```python
from build123d import *

# Parameters (mm, degrees)
F0_W      = 126.2549012899
F0_H      = 84.0705931187
F1_DEPTH  = 10
F2_W      = 119.4519400597
F2_H      = 78.4470066428
F3_DEPTH  = 9
F6_R      = 2.7574274492
F6_R_2    = 3.0881184617
F6_R_3    = 2.9865161703
F7_DEPTH  = 9.5
F5_R      = 3.0287162896
F8_DEPTH  = 9.5
F4_R      = 3.8384708655
F9_DEPTH  = 9.5
F10_R     = 3.132111717
F10_R_2   = 2.9916448853
F10_R_3   = 3.0367007185
F10_R_4   = 2.8900379759
F11_DEPTH = 9.5
F13_R     = 3.0036385534
F13_R_2   = 2.9794176667
F13_R_3   = 3.6399459422
F13_R_4   = 3.1255773117
F14_DEPTH = 9.5
F12_R     = 3.2154485225
F12_R_2   = 2.6789056155
F12_R_3   = 3.0133824395
F12_R_4   = 3.8856724273
F15_DEPTH = 9.5
F16_R     = 3.6323450942
F16_R_2   = 3.9223279678
F17_DEPTH = 9.5


# Not quite as in the source:
# - a feature names something its author has since deleted; it is built from what else it names


with BuildPart() as f1:
    # F0 (on Top) → F1 (new body)
    with BuildSketch(Plane.XY):
        Rectangle(F0_W, F0_H)
    extrude(amount=-F1_DEPTH)

    # F2 (on Top) → F3 (cut)
    with BuildSketch(Plane.XY):
        Rectangle(F2_W, F2_H)
    extrude(amount=-F3_DEPTH, mode=Mode.SUBTRACT)

    # F6 (on Top) → F7 (cut)
    with BuildSketch(Plane.XY):
        with Locations((16.5214389563, -8.0118775368)):
            Circle(F6_R)
        with Locations((-16.615998, -8.0534629524)):
            Circle(F6_R_2)
        with Locations((-16.615998, 8.0431699753)):
            Circle(F6_R_3)
    extrude(amount=-F7_DEPTH, mode=Mode.SUBTRACT)

    # F5 (on Top) → F8 (cut)
    with BuildSketch(Plane.XY):
        with Locations((16.5819376707, 7.8347064555)):
            Circle(F5_R)
    extrude(amount=-F8_DEPTH, mode=Mode.SUBTRACT)

    # F4 (on Top) → F9 (cut)
    with BuildSketch(Plane.XY):
        Circle(F4_R)
    extrude(amount=-F9_DEPTH, mode=Mode.SUBTRACT)

    # F10 (on face) → F11 (cut)
    with BuildSketch(Plane.XY):
        with Locations((29.441639781, 19.3310081959)):
            Circle(F10_R)
        with Locations((29.7522768378, -19.6110159159)):
            Circle(F10_R_2)
        with Locations((-29.6404287219, -19.6110159159)):
            Circle(F10_R_3)
        with Locations((-29.5161753893, 19.5709131658)):
            Circle(F10_R_4)
    extrude(amount=-F11_DEPTH, mode=Mode.SUBTRACT)

    # F13 (on Top) → F14 (cut)
    with BuildSketch(Plane.XY):
        with Locations((-34.714885056, 0)):
            Circle(F13_R)
        with Locations((35.1781696081, 0)):
            Circle(F13_R_2)
        with Locations((-51.6325049102, 0)):
            Circle(F13_R_3)
        with Locations((51.6923218966, 0)):
            Circle(F13_R_4)
    extrude(amount=-F14_DEPTH, mode=Mode.SUBTRACT)

    # F12 (on Top) → F15 (cut)
    with BuildSketch(Plane.XY):
        with Locations((-51.8871918321, 32.8838564456)):
            Circle(F12_R)
        with Locations((-51.9447661936, -32.4058681726)):
            Circle(F12_R_2)
        with Locations((51.5429228544, -32.7062048018)):
            Circle(F12_R_3)
        with Locations((51.7358258367, 31.9894589484)):
            Circle(F12_R_4)
    extrude(amount=-F15_DEPTH, mode=Mode.SUBTRACT)

    # F16 (on Top) → F17 (cut)
    with BuildSketch(Plane.XY):
        with Locations((0, 25.2807121724)):
            Circle(F16_R)
        with Locations((0, -27.0220451057)):
            Circle(F16_R_2)
    extrude(amount=-F17_DEPTH, mode=Mode.SUBTRACT)


solid = f1.part
```
CAD build for the part. Positions are in the model's coordinates, mm. A direction names the side the tool comes from. Round coordinates to 2 decimals unless told otherwise and drop trailing zeros. Write each loop counter-clockwise with the first axis right and the second up, starting at its lowest first coordinate (ties: lowest second). Pieces come first, ordered by that corner, then holes.
Item 1: Band-saw the part on B-B on z = -2.5. Write the cut outline in (x, y).
Filled in:
outline: (-63.13, -42.04) - (63.13, -42.04) - (63.13, 42.04) - (-63.13, 42.04) - close; hole (-59.73, -39.22) - (59.73, -39.22) - (59.73, 39.22) - (-59.73, 39.22) - close
Item 2: Drop flat-ended pins along their axis: pin 1 Ø3 at (x, y) = (17.5, 7) entering from +Z; pin 2 Ø6 at (x, y) = (16, -8) entering from +Z. Give the stop position or say it passes through.
Filled in:
pin 1: stops at z = -9.5
pin 2: stops at z = -9
Item 3: Band-saw the part on A-A on x = 0. Write the cut outline in (y, z).
Filled in:
outline: (-42.04, -10) - (42.04, -10) - (42.04, 0) - (39.22, 0) - (39.22, -9) - (28.91, -9) - (28.91, -9.5) - (21.65, -9.5) - (21.65, -9) - (3.84, -9) - (3.84, -9.5) - (-3.84, -9.5) - (-3.84, -9) - (-23.1, -9) - (-23.1, -9.5) - (-30.94, -9.5) - (-30.94, -9) - (-39.22, -9) - (-39.22, 0) - (-42.04, 0) - close
Item 4: Mould opens along Y. For faces 1 (the flat face through (63.127, -1, -5)), 2 (the cylindrical face through (-32.403, 19.698, -9.246)) say: released by +Y, released by -Y, zero draft, split by the parting line, or undercut.
Filled in:
face 1: zero draft
face 2: undercut
Item 5: Band-saw the part on D-D on x = -28.5. Write the cut outline in (y, z), then the cut area to 3 significant figures.
Filled in:
outline: (-42.04, -10) - (42.04, -10) - (42.04, 0) - (39.22, 0) - (39.22, -9) - (22.28, -9) - (22.28, -9.5) - (16.87, -9.5) - (16.87, -9) - (-16.8, -9) - (-16.8, -9.5) - (-22.43, -9.5) - (-22.43, -9) - (-39.22, -9) - (-39.22, 0) - (-42.04, 0) - close
area: 129 mm2
Item 6: Band-saw the part on C-C on y = 0. Write the cut outline in (x, z).
Filled in:
outline: (-63.13, -10) - (63.13, -10) - (63.13, 0) - (59.73, 0) - (59.73, -9) - (54.82, -9) - (54.82, -9.5) - (48.57, -9.5) - (48.57, -9) - (38.16, -9) - (38.16, -9.5) - (32.2, -9.5) - (32.2, -9) - (3.84, -9) - (3.84, -9.5) - (-3.84, -9.5) - (-3.84, -9) - (-31.71, -9) - (-31.71, -9.5) - (-37.72, -9.5) - (-37.72, -9) - (-47.99, -9) - (-47.99, -9.5) - (-55.27, -9.5) - (-55.27, -9) - (-59.73, -9) - (-59.73, 0) - (-63.13, 0) - close
Item 7: Tool access for faces 3 (the flat face through (-1, 1, -10)), 4 (the flat face through (-1, -39.224, -4)): list every direction of +Z, -Z, +X, -X, +Y, -Y with a clear straight run to the whole face (end or side of a thin tool).
Filled in:
face 3: -Z, +X, -X, +Y, -Y
face 4: +Z
Item 8: Drill centre lines: L1, parallel to Y at x = 0, z = -9.4; L2, parallel to Y at x = 50, z = -2.75; L3, parallel to X at y = 6, z = -6. Where is each one in solid material? Low to high.
Filled in:
L1: y = -42.04 to -30.94, -23.1 to -3.84, 3.84 to 21.65, 28.91 to 42.04
L2: y = -42.04 to -39.22, 39.22 to 42.04
L3: x = -63.13 to -59.73, 59.73 to 63.13
